```python
from build123d import *

# Parameters (mm, degrees)
SALIENTE_EXTRUIR1_DEPTH = 2
CORTAR_EXTRUIR1_START   = -2
CROQUIS2_R              = 2.2499999999999543
CROQUIS2_R_2            = 2.2499999999999525
CORTAR_EXTRUIR1_DEPTH   = 2
SALIENTE_EXTRUIR2_DEPTH = 25
REDONDEO1_R             = 5
REDONDEO2_R             = 2.5
CORTAR_EXTRUIR2_DEPTH   = 150
REDONDEO3_R             = 1
REDONDEO4_R             = 2


with BuildPart() as part:
    # Croquis1 → Saliente-Extruir1 (new body)
    with BuildSketch(Plane(origin=(-11.563192139466418, 0, 0), x_dir=(0, 0, -1), z_dir=(1, 0, 0))):
        with BuildLine():
            Line((-487.50000000000006, 61.20002010491962), (-487.50000000000006, 76.20002010491963))
            ThreePointArc((-487.50000000000006, 76.20002010491963), (-485.5828732625374, 80.13650234762473), (-481.3016430211471, 81.05429044671504))
            ThreePointArc((-481.3016430211471, 81.05429044671504), (-454.3213610685335, 75.37256140046077), (-427.01376608968735, 71.56297931460594))
            ThreePointArc((-427.01376608968735, 71.56297931460594), (-419.99597330488047, 71.19728769059765), (-412.9781919309264, 71.56319822849083))
            ThreePointArc((-412.9781919309264, 71.56319822849083), (-385.6746727662309, 75.37294023507445), (-358.6984109055162, 81.05427713370786))
            ThreePointArc((-358.6984109055162, 81.05427713370786), (-354.4171486029636, 80.13651947158925), (-352.50000000000006, 76.20002010491963))
            Line((-352.50000000000006, 76.20002010491963), (-352.50000000000006, 61.20002010491962))
            ThreePointArc((-352.50000000000006, 61.20002010491962), (-354.41718437935106, 57.26349272039885), (-358.698499139633, 56.3457848600743))
            ThreePointArc((-358.698499139633, 56.3457848600743), (-385.67550243814526, 62.027759813352475), (-412.9798133969885, 65.8380287540453))
            ThreePointArc((-412.9798133969885, 65.8380287540453), (-420, 66.20405869011226), (-427.02018660301155, 65.83802875404524))
            ThreePointArc((-427.02018660301155, 65.83802875404524), (-454.3244975618549, 62.027759813352304), (-481.3015008603671, 56.34578486007424))
            ThreePointArc((-481.3015008603671, 56.34578486007424), (-485.5828156206491, 57.2634927203988), (-487.50000000000006, 61.20002010491962))
        make_face()
    extrude(amount=SALIENTE_EXTRUIR1_DEPTH)

    # Croquis2 → Cortar-Extruir1 (cut)
    with BuildSketch(Plane(origin=(-9.563192139466418, 0, 0), x_dir=(0, 0, -1), z_dir=(1, 0, 0)).offset(CORTAR_EXTRUIR1_START)):
        with Locations((-357.50000000000006, 61.20002010491962)):
            Circle(CROQUIS2_R)
        with Locations((-482.50000000000006, 61.20002010491962)):
            Circle(CROQUIS2_R)
        with Locations((-482.50000000000006, 76.20002010491963)):
            Circle(CROQUIS2_R_2)
        with Locations((-357.50000000000006, 76.20002010491963)):
            Circle(CROQUIS2_R_2)
        with BuildLine():
            Line((-471.00000000000006, 74.70002010491963), (-471.00000000000006, 78.65520707766471))
            ThreePointArc((-471.00000000000006, 78.65520707766471), (-468.00242565546085, 78.0108082929201), (-465, 77.3894050999363))
            Line((-465, 77.3894050999363), (-465, 74.70002010491963))
            ThreePointArc((-465, 74.70002010491963), (-468, 71.70002010491957), (-471.00000000000006, 74.70002010491963))
        make_face()
        with BuildLine():
            Line((-471.00000000000006, 62.70002010491962), (-471.00000000000006, 58.745154173439786))
            ThreePointArc((-471.00000000000006, 58.745154173439786), (-468.0024260238705, 59.38964522535156), (-465, 60.011140542750915))
            Line((-465, 60.011140542750915), (-465, 62.70002010491962))
            ThreePointArc((-465, 62.70002010491962), (-468, 65.70002010491962), (-471.00000000000006, 62.70002010491962))
        make_face()
        with BuildLine():
            Line((-375.00000000000006, 74.70002010492064), (-375.00000000000006, 77.3892133718565))
            ThreePointArc((-375.00000000000006, 77.3892133718565), (-371.9975742047899, 78.0106515107218), (-369.00000000000006, 78.65508529549625))
            Line((-369.00000000000006, 78.65508529549625), (-369.00000000000006, 74.70002010492064))
            ThreePointArc((-369.00000000000006, 74.70002010492064), (-372.00000000000006, 71.70002010492064), (-375.00000000000006, 74.70002010492064))
        make_face()
        with BuildLine():
            Line((-375.00000000000006, 62.700020104920625), (-375.00000000000006, 60.01114054275103))
            ThreePointArc((-375.00000000000006, 60.01114054275103), (-371.9975739761297, 59.38964522535167), (-369.00000000000006, 58.74515417343995))
            Line((-369.00000000000006, 58.74515417343995), (-369.00000000000006, 62.700020104920625))
            ThreePointArc((-369.00000000000006, 62.700020104920625), (-372.00000000000006, 65.70002010492063), (-375.00000000000006, 62.700020104920625))
        make_face()
    extrude(amount=CORTAR_EXTRUIR1_DEPTH, mode=Mode.SUBTRACT)

    # Croquis3 → Saliente-Extruir2 (add)
    with BuildSketch(Plane(origin=(-9.563192139466418, 0, 0), x_dir=(0, 0, -1), z_dir=(1, 0, 0))):
        with BuildLine():
            Line((-441.5, 73.34478345263268), (-441.5, 64.0564693169966))
            ThreePointArc((-441.5, 64.0564693169966), (-439.500688579451, 64.33441688299206), (-437.50000000000006, 64.60227172023619))
            Line((-437.50000000000006, 64.60227172023619), (-437.50000000000006, 72.79909943134032))
            ThreePointArc((-437.50000000000006, 72.79909943134032), (-439.5006884273723, 73.06689509761537), (-441.5, 73.34478345263268))
        make_face()
        with BuildLine():
            Line((-402.51863522626155, 64.60471833694513), (-402.5055085249573, 72.7978713543057))
            ThreePointArc((-402.5055085249573, 72.7978713543057), (-400.5049833223084, 73.06563889552336), (-398.50583471542444, 73.34349747494228))
            Line((-398.50583471542444, 73.34349747494228), (-398.52070927713964, 64.05940108438512))
            ThreePointArc((-398.52070927713964, 64.05940108438512), (-400.5189846456923, 64.33710080901727), (-402.51863522626155, 64.60471833694513))
        make_face()
    extrude(amount=SALIENTE_EXTRUIR2_DEPTH)

    # Redondeo1
    # the kernel refuses this fillet: 5 mm, written as the material it takes off along each edge
    with BuildSketch(Plane(origin=(15.436807860533582, -331.99303473076, 454.57843031070206), x_dir=(0, 0.9852688696585968, -0.17101243955242207), z_dir=(0, -0.17101243955242207, -0.9852688696585968))) as redondeo1_piece_1:
        with BuildLine():
            CenterArc((400.0000000032307 + REDONDEO1_R, -REDONDEO1_R), REDONDEO1_R, 90, 90)
            Line((400.0000000032307 + REDONDEO1_R, 0), (400.0000000032307, 0))
            Line((400.0000000032307, 0), (400.0000000032307, -REDONDEO1_R))
        make_face()
    revolve(axis=Axis((15.436807860533582, -331.99303473076, 454.57843031070206), (1, 0, 0)), revolution_arc=4.158952056224013, mode=Mode.SUBTRACT)
    with BuildSketch(Plane(origin=(15.436807860533582, 469.39483943387535, 454.5712833464088), x_dir=(0, -0.9950753091360283, -0.09912178947051785), z_dir=(0, -0.09912178947051785, 0.9950753091360283))) as redondeo1_piece_2:
        with BuildLine():
            CenterArc((399.9999999970836 + REDONDEO1_R, -REDONDEO1_R), REDONDEO1_R, 90, 90)
            Line((399.9999999970836 + REDONDEO1_R, 0), (399.9999999970836, 0))
            Line((399.9999999970836, 0), (399.9999999970836, -REDONDEO1_R))
        make_face()
    revolve(axis=Axis((15.436807860533582, 469.39483943387535, 454.5712833464088), (1, 0, 0)), revolution_arc=4.159206104487057, mode=Mode.SUBTRACT)
    with BuildSketch(Plane(origin=(15.436807860533582, 469.3959177926432, 385.43308471259814), x_dir=(0, -0.9950750240944541, 0.09912465093719791), z_dir=(0, -0.09912465093719791, -0.9950750240944541))) as redondeo1_piece_3:
        with BuildLine():
            CenterArc((400.0000000023156 + REDONDEO1_R, REDONDEO1_R), REDONDEO1_R, 180, 90)
            Line((400.0000000023156 + REDONDEO1_R, 0), (400.0000000023156, 0))
            Line((400.0000000023156, 0), (400.0000000023156, REDONDEO1_R))
        make_face()
    revolve(axis=Axis((15.436807860533582, 469.3959177926432, 385.43308471259814), (-1, 0, 0)), revolution_arc=4.159253520630329, mode=Mode.SUBTRACT)
    with BuildSketch(Plane(origin=(15.436807860533582, -331.99303472992847, 385.4215696894115), x_dir=(0, 0.9852599261695624, 0.1710639584610054), z_dir=(0, -0.1710639584610054, 0.9852599261695624))) as redondeo1_piece_4:
        with BuildLine():
            CenterArc((400.00000000239186 + REDONDEO1_R, REDONDEO1_R), REDONDEO1_R, 180, 90)
            Line((400.00000000239186 + REDONDEO1_R, 0), (400.00000000239186, 0))
            Line((400.00000000239186, 0), (400.00000000239186, REDONDEO1_R))
        make_face()
    revolve(axis=Axis((15.436807860533582, -331.99303472992847, 385.4215696894115), (-1, 0, 0)), revolution_arc=4.159255812959428, mode=Mode.SUBTRACT)

    # Redondeo2
    redondeo2_edges = [part.edges().sort_by_distance(p)[0] for p in [
        (-9.563192139466418, 68.70062638481464, 441.5),
        (-9.563192139466418, 68.70068557578826, 437.50000000000006),
        (-9.563192139466418, 68.7014492796637, 398.51327199628207),
        (-9.563192139466418, 68.70129484562541, 402.5120718756094),
    ]]
    fillet(redondeo2_edges, radius=REDONDEO2_R)

    # Croquis4 → Cortar-Extruir2 (cut)
    with BuildSketch(Plane.XY.offset(441.5)):
        with BuildLine():
            Line((9.936807860533582, 71.84478345263268), (-6.063192139466418, 71.84478345263268))
            Line((-6.063192139466418, 71.84478345263268), (-6.063192139466418, 65.5564693169966))
            Line((-6.063192139466418, 65.5564693169966), (9.936807860533582, 65.55646931699658))
            ThreePointArc((9.936807860533582, 65.55646931699658), (13.080964928351639, 68.70062638481464), (9.936807860533582, 71.84478345263268))
        make_face()
    extrude(amount=-CORTAR_EXTRUIR2_DEPTH, mode=Mode.SUBTRACT)

    # Redondeo3
    redondeo3_edges = [part.edges().sort_by_distance(p)[0] for p in [
        (-6.063192139466418, 65.5564693169966, 439.5),
        (-6.063192139466418, 65.5564693169966, 400.51771055769314),
        (-6.063192139466418, 71.84478345263268, 439.5),
        (-6.063192139466418, 71.84478345263268, 400.5076357035813),
    ]]
    fillet(redondeo3_edges, radius=REDONDEO3_R)

    # Redondeo4
    redondeo4_edges = [part.edges().sort_by_distance(p)[0] for p in [
        (-10.563192139466418, 58.74515417343996, 369.00000000000006),
        (-10.563192139466418, 60.011140542751036, 375.00000000000006),
        (-10.563192139466418, 77.38921337185644, 375),
        (-10.563192139466418, 78.6550852954962, 369.00000000000006),
        (-10.563192139466418, 60.01114054275092, 465),
        (-10.563192139466418, 58.74515417343982, 471.00000000000006),
        (-10.563192139466418, 78.6552070776647, 471.00000000000006),
        (-10.563192139466418, 77.38940509993628, 465),
    ]]
    fillet(redondeo4_edges, radius=REDONDEO4_R)


solid = part.part
```
Could you check a few things on this model? Use its own coordinates, in mm. A direction names the side the tool comes from. Coordinates: 2 decimals unless noted, no trailing zeros. Write each loop counter-clockwise with the first axis right and the second up, starting at its lowest first coordinate (ties: lowest second). Pieces come first, ordered by that corner, then holes. Notation, with made-up numbers: (71.25, 22.25) -> (97.25, 22.25) arc R27 cw to (97.25, 43.25) -> close; hole circle Ø10 at (79.25, 56.5). An arc over 180 degrees is marked (long way). Write item = value, one per line. Start each with the question number.
(1) We'd pull the mould along X, two halves only. Please class faces 4 (the face through (-9.563, 69, 420)), 5 (the face through (5, 72, 437.5)), 6 (the face through (13.08, 68.63, 439.53)): released by +X, released by -X, zero draft, split by the parting line, or undercut.
(2) I want a section at C-C (z = 372). Please give me the cut outline in (x, y), plus the area to 3 significant figures.
(3) I need wall thicknesses on line 1 (Y direction, x = -10.65, z = 357.5); line 2 (Z direction, x = 3.5, y = 72.5); line 3 (X direction, y = 59.25, z = 367). Which ranges of each line are inside material? Lowest first, please. Write a range as [from, to].
(4) I want a section at A-A (x = 7). Please give me the cut outline in (y, z), plus the area to 3 significant figures.
(5) Will these pins go through, and if not, where does the flat tip stop? pin 1 (5 mm diameter, centred on y = 67, z = 436, fed in from +X); pin 2 (1.5 mm diameter, centred on x = 0, y = 75.5, fed in from -Z); pin 3 (6 mm diameter, centred on x = 12.5, y = 67, fed in from +Z); pin 4 (8.5 mm diameter, centred on y = 67.5, z = 426, fed in from +X).
(6) Which directions (+Z, -Z, +X, -X, +Y, -Y) give clear straight access to the entire face, cutting with the end or side of a thin tool? Please do faces 1 (the face through (-5.5, 64.15, 440.84)), 2 (the face through (-9.563, 69, 470)), 3 (the face through (3, 71.845, 401)).
(7) I want a section at B-B (z = 482.5). Please give me the cut outline in (x, y), plus the area to 3 significant figures.
(8) I want a section at D-D (z = 424). Please give me the cut outline in (x, y).
Result set:
q1.face_4 = released by +X
q1.face_5 = zero draft
q1.face_6 = undercut
q2.outline = (-11.56, 65.7) -> (-9.56, 65.7) -> (-9.56, 71.7) -> (-11.56, 71.7) -> close
q2.area = 12.0 mm2
q3.line_1 = [56.2, 58.95], [63.45, 73.95], [78.45, 81.2]
q3.line_2 = [398.51, 402.51], [437.5, 441.5]
q3.line_3 = [-11.56, -9.56]
q4.outline = (64.06, 398.52) -> (65.56, 398.52) -> (65.56, 402.52) -> (64.6, 402.52) arc R400 cw to start; (64.06, 441.5) arc R400 cw to (64.6, 437.5) -> (65.56, 437.5) -> (65.56, 441.5) -> close; (71.84, 398.51) -> (73.34, 398.51) arc R400 cw to (72.8, 402.51) -> (71.84, 402.51) -> close; (71.84, 437.5) -> (72.8, 437.5) arc R400 cw to (73.34, 441.5) -> (71.84, 441.5) -> close
q4.area = 19.6 mm2
q5.pin_1 = 15.36
q5.pin_2 = through
q5.pin_3 = 441.5
q5.pin_4 = -9.56
q6.face_1 = +X, -X, -Y
q6.face_2 = +Z, +X, +Y, -Y
q6.face_3 = +Z, -Z
q7.outline = (-11.56, 56.2) -> (-9.56, 56.2) -> (-9.56, 58.95) -> (-11.56, 58.95) -> close; (-11.56, 63.45) -> (-9.56, 63.45) -> (-9.56, 73.95) -> (-11.56, 73.95) -> close; (-11.56, 78.45) -> (-9.56, 78.45) -> (-9.56, 81.2) -> (-11.56, 81.2) -> close
q7.area = 32.0 mm2
q8.outline = (-11.56, 66.09) -> (-9.56, 66.09) -> (-9.56, 71.32) -> (-11.56, 71.32) -> close
